```python
from build123d import *

# Parameters (mm, degrees)
BOSS_EXTRUDE1_DEPTH = 6
SKETCH2_R           = 1.1
CUT_EXTRUDE1_DEPTH  = 2


with BuildPart() as part:
    # Sketch1 → Boss-Extrude1 (new body)
    with BuildSketch(Plane(origin=(0, 0, 0), x_dir=(1, 0, 0), z_dir=(0, 1, 0))):
        Polygon((13, 0), (13, -4), (27, -4), (27, 0), (43, 0), (43, 25), (40, 25), (40, 3), (0, 3), (0, 25), (-3, 25), (-3, 0), align=None)
        Polygon((25, -2), (20, -2), (15, -2), (15, 0), (25, 0), align=None, mode=Mode.SUBTRACT)
    extrude(amount=BOSS_EXTRUDE1_DEPTH)

    # Sketch2 → Cut-Extrude1 (cut)
    with BuildSketch(Plane.XY.offset(4)):
        with Locations((20, 3)):
            Circle(SKETCH2_R)
    extrude(amount=-CUT_EXTRUDE1_DEPTH, mode=Mode.SUBTRACT)


solid = part.part
```
Geometry check sheet. Reference: the model listing, model coordinates, mm. A direction names the side the tool comes from. Round coordinates to 2 decimals unless told otherwise and drop trailing zeros. Order: outer loops, then holes, each group sorted by start corner. A loop starts at its lowest first (then second) coordinate and runs counter-clockwise, first axis right, second up. Notation, with made-up numbers: (38.5, 28.5) - (52.5, 28.5) arc R8 ccw to (52.5, 37.5) - close; hole circle Ø10 at (85, 36). An arc over 180 degrees is marked (long way). Use a Markdown table: item, result. Add a question column.
1) Section check A-A (y = 4.6). Record the cut outline in (x, z).
2) Section check B-B (z = -17). Record the cut outline in (x, y).
3) Thickness scan on line 1 along Y through (x, z) = (20, 2.4); line 2 along X through (y, z) = (1.5, -7); line 3 along Z through (x, y) = (24.5, 4.3). Record the ranges inside material, lowest first.
4) Mould release check, pull along Y, two halves, no side actions. Record for faces 4 (the flat face through (22, 6, -2)), 5 (the flat face through (-1, 3, -25)), 6 (the cylindrical face through (18.9, 3, 3)): released by +Y, released by -Y, zero draft, split by the parting line, or undercut.
5) Gauge pin test, flat ends, axial feed: P1, Ø3, axis at y = 2.5, z = 3, coming from the -X side; P2, Ø2, axis at x = 20, y = 3, coming from the -Z side; P3, Ø3, axis at x = 38.5, y = 4, coming from the +Z side. Record the tip position at first contact, or that the pin passes through.
6) Set-up check for faces 1 (the flat face through (0, 3, -14)), 2 (the flat face through (21, 2, 2)), 3 (the flat face through (13, 3, 2)): record each of +Z, -Z, +X, -X, +Y, -Y from which the full face is reachable in a straight line by a thin tool's end or side.
7) Section check D-D (x = 1.5). Record the cut outline in (y, z), then the cut area to 3 significant figures.
8) Section check C-C (x = 20). Record the cut outline in (y, z), then the cut area to 3 significant figures.
Established:
| question | item | result |
|---|---|---|
| 1 | outline | (-3, -25) - (0, -25) - (0, -3) - (40, -3) - (40, -25) - (43, -25) - (43, 0) - (27, 0) - (27, 4) - (13, 4) - (13, 0) - (-3, 0) - close; hole (15, 0) - (25, 0) - (25, 2) - (15, 2) - close |
| 2 | outline | (-3, 0) - (0, 0) - (0, 6) - (-3, 6) - close; (40, 0) - (43, 0) - (43, 6) - (40, 6) - close |
| 3 | line 1 | 0 to 1.9, 4.1 to 6 |
| 3 | line 2 | -3 to 0, 40 to 43 |
| 3 | line 3 | -3 to 0, 2 to 4 |
| 4 | face 4 | released by +Y |
| 4 | face 5 | zero draft |
| 4 | face 6 | undercut |
| 5 | P1 | x = 13 |
| 5 | P2 | z = -3 |
| 5 | P3 | z = 0 |
| 6 | face 1 | -Z, +Y, -Y |
| 6 | face 2 | +Y, -Y |
| 6 | face 3 | +Z, -X, +Y, -Y |
| 7 | outline | (0, -3) - (6, -3) - (6, 0) - (0, 0) - close |
| 7 | area | 18.0 mm2 |
| 8 | outline | (0, -3) - (6, -3) - (6, 0) - (0, 0) - close; (0, 2) - (1.9, 2) - (1.9, 4) - (0, 4) - close; (4.1, 2) - (6, 2) - (6, 4) - (4.1, 4) - close |
| 8 | area | 25.6 mm2 |
